```python
from build123d import *

# Parameters (mm, degrees)
BOSS_EXTRUDE1_DEPTH      = 2
BOSS_EXTRUDE2_DEPTH      = 1.7
BOSS_EXTRUDE2_DEPTH_BACK = 1.7
BOSS_EXTRUDE3_DEPTH      = 1.7
BOSS_EXTRUDE3_DEPTH_BACK = 1.7
BOSS_EXTRUDE4_DEPTH      = 1.7
BOSS_EXTRUDE4_DEPTH_BACK = 1.7
BOSS_EXTRUDE5_DEPTH      = 1.7
BOSS_EXTRUDE5_DEPTH_BACK = 1.7
SKETCH6_W                = 38.6
SKETCH6_H                = 47.5
CUT_EXTRUDE1_DEPTH       = 4
BOSS_EXTRUDE6_DEPTH      = 3.8
BOSS_EXTRUDE7_DEPTH      = 3.8
CUT_EXTRUDE2_DEPTH       = 20
CUT_EXTRUDE2_DEPTH_BACK  = 20
CUT_EXTRUDE3_DEPTH       = 11.15
CUT_EXTRUDE3_DEPTH_BACK  = 11.15
CUT_EXTRUDE4_DEPTH       = 11.15
CUT_EXTRUDE4_DEPTH_BACK  = 11.15
CUT_EXTRUDE5_DEPTH       = 16
CUT_EXTRUDE5_DEPTH_BACK  = 16
CUT_EXTRUDE6_DEPTH       = 16
CUT_EXTRUDE6_DEPTH_BACK  = 16


with BuildPart() as part:
    # Sketch1 → Boss-Extrude1 (new body)
    with BuildSketch(Plane.XY):
        with BuildLine():
            Line((-14.3, 18.25), (-14.3, -18.25))
            ThreePointArc((-14.3, -18.25), (-14.153553391, -18.603553391), (-13.8, -18.75))
            Line((-13.8, -18.75), (13.8, -18.75))
            ThreePointArc((13.8, -18.75), (14.153553391, -18.603553391), (14.3, -18.25))
            Line((14.3, -18.25), (14.3, 18.25))
            ThreePointArc((14.3, 18.25), (14.153553391, 18.603553391), (13.8, 18.75))
            Line((13.8, 18.75), (-13.8, 18.75))
            ThreePointArc((-13.8, 18.75), (-14.153553391, 18.603553391), (-14.3, 18.25))
        make_face()
    extrude(amount=BOSS_EXTRUDE1_DEPTH)

    # Sketch2 → Boss-Extrude2 (add, two sides)
    with BuildSketch(Plane.XY) as boss_extrude2_sk:
        with BuildLine():
            Line((-13.1, 12.5), (-10.1, 12.5))
            ThreePointArc((-10.1, 12.5), (-9.35, 13.25), (-10.1, 14))
            Line((-10.1, 14), (-13.1, 14))
            Line((-13.1, 14), (-13.1, 12.5))
        make_face()
    extrude(amount=BOSS_EXTRUDE2_DEPTH)
    extrude(boss_extrude2_sk.sketch, amount=-BOSS_EXTRUDE2_DEPTH_BACK)

    # Sketch3 → Boss-Extrude3 (add, two sides)
    with BuildSketch(Plane.XY) as boss_extrude3_sk:
        with BuildLine():
            Line((10.1, -14), (13.1, -14))
            Line((13.1, -14), (13.1, -12.5))
            Line((13.1, -12.5), (10.1, -12.5))
            ThreePointArc((10.1, -12.5), (9.35, -13.25), (10.1, -14))
        make_face()
    extrude(amount=BOSS_EXTRUDE3_DEPTH)
    extrude(boss_extrude3_sk.sketch, amount=-BOSS_EXTRUDE3_DEPTH_BACK)

    # Sketch4 → Boss-Extrude4 (add, two sides)
    with BuildSketch(Plane.XY) as boss_extrude4_sk:
        with BuildLine():
            Line((-13.1, -12.5), (-13.1, -14))
            Line((-13.1, -14), (-10.1, -14))
            ThreePointArc((-10.1, -14), (-9.35, -13.25), (-10.1, -12.5))
            Line((-10.1, -12.5), (-13.1, -12.5))
        make_face()
    extrude(amount=BOSS_EXTRUDE4_DEPTH)
    extrude(boss_extrude4_sk.sketch, amount=-BOSS_EXTRUDE4_DEPTH_BACK)

    # Sketch5 → Boss-Extrude5 (add, two sides)
    with BuildSketch(Plane.XY) as boss_extrude5_sk:
        with BuildLine():
            Line((10.1, 12.5), (13.1, 12.5))
            Line((13.1, 12.5), (13.1, 14))
            Line((13.1, 14), (10.1, 14))
            ThreePointArc((10.1, 14), (9.35, 13.25), (10.1, 12.5))
        make_face()
    extrude(amount=BOSS_EXTRUDE5_DEPTH)
    extrude(boss_extrude5_sk.sketch, amount=-BOSS_EXTRUDE5_DEPTH_BACK)

    # Sketch6 → Cut-Extrude1 (cut)
    with BuildSketch(Plane.XY.offset(-3)):
        Rectangle(SKETCH6_W, SKETCH6_H)
        with BuildLine():
            Line((-14.3, -4.045), (-11.298993595, -4.045))
            ThreePointArc((-11.298993595, -4.045), (-10.927421183, -4.210434697), (-10.801732648, -4.597264232))
            Line((-10.801732648, -4.597264232), (-11.79, -14))
            Line((-11.79, -14), (-8.55, -14))
            ThreePointArc((-8.55, -14), (-8.196446609, -14.146446609), (-8.05, -14.5))
            Line((-8.05, -14.5), (-8.05, -18.75))
            Line((-8.05, -18.75), (8.05, -18.75))
            Line((8.05, -18.75), (8.05, -14.5))
            ThreePointArc((8.05, -14.5), (8.196446609, -14.146446609), (8.55, -14))
            Line((8.55, -14), (11.79, -14))
            Line((11.79, -14), (10.801732648, -4.597264232))
            ThreePointArc((10.801732648, -4.597264232), (10.927421183, -4.210434697), (11.298993595, -4.045))
            Line((11.298993595, -4.045), (14.3, -4.045))
            Line((14.3, -4.045), (14.3, 4.045))
            Line((14.3, 4.045), (11.298993595, 4.045))
            ThreePointArc((11.298993595, 4.045), (10.927421183, 4.210434697), (10.801732648, 4.597264232))
            Line((10.801732648, 4.597264232), (11.79, 14))
            Line((11.79, 14), (8.55, 14))
            ThreePointArc((8.55, 14), (8.196446609, 14.146446609), (8.05, 14.5))
            Line((8.05, 14.5), (8.05, 18.75))
            Line((8.05, 18.75), (-8.05, 18.75))
            Line((-8.05, 18.75), (-8.05, 14.5))
            ThreePointArc((-8.05, 14.5), (-8.196446609, 14.146446609), (-8.55, 14))
            Line((-8.55, 14), (-11.79, 14))
            Line((-11.79, 14), (-10.801732648, 4.597264232))
            ThreePointArc((-10.801732648, 4.597264232), (-10.927421183, 4.210434697), (-11.298993595, 4.045))
            Line((-11.298993595, 4.045), (-14.3, 4.045))
            Line((-14.3, 4.045), (-14.3, -4.045))
        make_face(mode=Mode.SUBTRACT)
    extrude(amount=CUT_EXTRUDE1_DEPTH, mode=Mode.SUBTRACT)

    # Sketch7 → Boss-Extrude6 (add)
    with BuildSketch(Plane.XY.offset(-3.6)):
        Polygon((12.36, -4.002188077), (13.547735768, -15.302739052), (14.1, -15.8), (15.35, -15.8), (14.779051792, -11.15), (14.04, -11.15), (14.04, 11.15), (14.779051792, 11.15), (15.35, 15.8), (14.1, 15.8), (13.547735768, 15.302739052), (12.36, 4.002188077), align=None)
    extrude(amount=BOSS_EXTRUDE6_DEPTH)

    # Sketch8 → Boss-Extrude7 (add)
    with BuildSketch(Plane.XY.offset(-3.6)):
        Polygon((-15.35, -15.8), (-14.1, -15.8), (-13.547735768, -15.302739052), (-12.36, -4.002188077), (-12.36, 4.002188077), (-13.547735768, 15.302739052), (-14.1, 15.8), (-15.35, 15.8), (-14.779051792, 11.15), (-14.04, 11.15), (-14.04, -11.15), (-14.779051792, -11.15), align=None)
    extrude(amount=BOSS_EXTRUDE7_DEPTH)

    # Sketch9 → Cut-Extrude2 (cut, two sides)
    with BuildSketch(Plane(origin=(0, 0, 0), x_dir=(0, 0, -1), z_dir=(1, 0, 0))) as cut_extrude2_sk:
        Polygon((2.395156371, -15.8), (8.5, -15.8), (8.5, 15.8), (2.395156371, 15.8), (3.5, 0), align=None)
    extrude(amount=CUT_EXTRUDE2_DEPTH, mode=Mode.SUBTRACT)
    extrude(cut_extrude2_sk.sketch, amount=-CUT_EXTRUDE2_DEPTH_BACK, mode=Mode.SUBTRACT)

    # Sketch10 → Cut-Extrude3 (cut, two sides)
    with BuildSketch(Plane(origin=(0, 0, 0), x_dir=(1, 0, 0), z_dir=(0, 1, 0))) as cut_extrude3_sk:
        Polygon((13.602556682, 4), (14.04, -1), (14.3, -1), (14.3, 4), align=None)
    extrude(amount=CUT_EXTRUDE3_DEPTH, mode=Mode.SUBTRACT)
    extrude(cut_extrude3_sk.sketch, amount=-CUT_EXTRUDE3_DEPTH_BACK, mode=Mode.SUBTRACT)

    # Sketch11 → Cut-Extrude4 (cut, two sides)
    with BuildSketch(Plane(origin=(0, 0, 0), x_dir=(1, 0, 0), z_dir=(0, 1, 0))) as cut_extrude4_sk:
        Polygon((-14.3, 4), (-14.3, -1), (-14.04, -1), (-13.602556682, 4), align=None)
    extrude(amount=CUT_EXTRUDE4_DEPTH, mode=Mode.SUBTRACT)
    extrude(cut_extrude4_sk.sketch, amount=-CUT_EXTRUDE4_DEPTH_BACK, mode=Mode.SUBTRACT)

    # Sketch12 → Cut-Extrude5 (cut, two sides)
    with BuildSketch(Plane(origin=(0, 0, 0), x_dir=(1, 0, 0), z_dir=(0, 1, 0))) as cut_extrude5_sk:
        Polygon((12.35, 4.8), (12.35, 4.675260778), (15.35, 1.1), (15.35, 0.6), (14.375049256, 0.428089879), (14.43, -0.2), (17.35, -0.2), (17.35, 4.8), align=None)
    extrude(amount=CUT_EXTRUDE5_DEPTH, mode=Mode.SUBTRACT)
    extrude(cut_extrude5_sk.sketch, amount=-CUT_EXTRUDE5_DEPTH_BACK, mode=Mode.SUBTRACT)

    # Sketch13 → Cut-Extrude6 (cut, two sides)
    with BuildSketch(Plane(origin=(0, 0, 0), x_dir=(1, 0, 0), z_dir=(0, 1, 0))) as cut_extrude6_sk:
        Polygon((-17.35, 4.8), (-17.35, -0.2), (-14.43, -0.2), (-14.375049256, 0.428089879), (-15.35, 0.6), (-15.35, 1.1), (-12.35, 4.675260778), (-12.35, 4.8), align=None)
    extrude(amount=CUT_EXTRUDE6_DEPTH, mode=Mode.SUBTRACT)
    extrude(cut_extrude6_sk.sketch, amount=-CUT_EXTRUDE6_DEPTH_BACK, mode=Mode.SUBTRACT)


solid = part.part
```
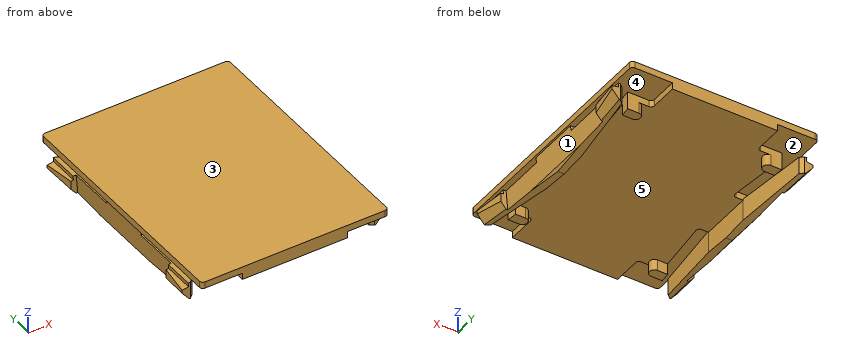
The model under review builds one solid part; all positions refer to its coordinate system, in mm. Face numbers are marked on the shaded views. A direction names the side the tool comes from. Coordinates: 2 decimals unless noted, no trailing zeros. Write each loop counter-clockwise with the first axis right and the second up, starting at its lowest first coordinate (ties: lowest second). Pieces come first, ordered by that corner, then holes. Notation, with made-up numbers: (-16, 6.5) - (11, 6.5) arc R6 cw to (11, 16.5) - close; hole circle Ø9 at (49.25, 25). An arc over 180 degrees is marked (long way). Answer in a Markdown table with one row per item. Add a question column.
Q1. To check wall thickness, follow line 1 along X through (y, z) = (-13, -0.6); line 2 along Y through (x, z) = (11, -0.15); line 3 along Z through (x, y) = (0, 1). State the ranges of each line that lie inside material, in increasing order. Write a range as from..to.
Q2. Consider section B-B on z = 1.4. Give the boundary of the cut face in (x, y).
Q3. Consider section C-C on x = -7.5. Give the boundary of the cut face in (y, z).
Q4. For the marked faces 1 and 2, list the 3-axis set-ups (+Z, -Z, +X, -X, +Y, -Y) from which the entire face can be reached by the end or side of a thin tool; tool diameter is ignored.
Q5. Consider section D-D on y = 13.25. Give the boundary of the cut face in (x, z), then the cut area to 3 significant figures.
Q6. Draft analysis for pull direction Z (two halves, no side actions). For the marked faces 3, 4 and 5, state which applies: +Z half, -Z half, draft (parallel to the pull), parting line (faces both ways), or undercut.
Q7. Clearance check with flat-ended pins moving along their axes: pin 1 (1 mm diameter, centred on y = -5, z = -1.5, fed in from +X) (3 decimals); pin 2 (0.5 mm diameter, centred on y = -17, z = 0.5, fed in from -X); pin 3 (0.6 mm diameter, centred on x = 15, z = -0.5, fed in from -Y); pin 4 (3 mm diameter, centred on x = 9.5, z = 0, fed in from +Y). State where each tip first meets the part, or that it passes through.
Q8. Consider section A-A on y = 8. Give the boundary of the cut face in (x, z), then the cut area to 3 significant figures.
Answers below:
| question | item | result |
|---|---|---|
| 1 | line 1 | -15.01..-13.31, -11.68..-9.39, 9.39..11.68, 13.31..15.01 |
| 1 | line 2 | -14..-12.5, 12.5..14 |
| 1 | line 3 | 0..2 |
| 2 | outline | (-14.3, -18.25) arc R0.5 ccw to (-13.8, -18.75) - (13.8, -18.75) arc R0.5 ccw to (14.3, -18.25) - (14.3, 18.25) arc R0.5 ccw to (13.8, 18.75) - (-13.8, 18.75) arc R0.5 ccw to (-14.3, 18.25) - close |
| 3 | outline | (-18.75, 0) - (18.75, 0) - (18.75, 2) - (-18.75, 2) - close |
| 4 | face 1 | -Z, +X |
| 4 | face 2 | -X |
| 5 | outline | (-15.04, -1.47) - (-14.11, -2.57) - (-13.33, -2.57) - (-13.33, 0.2) - (-14.43, 0.2) - (-14.38, -0.43) - (-15.04, -0.54) - close; (-14.3, 1) - (-11.71, 1) - (-11.71, -1.7) - (-9.35, -1.7) - (-9.35, 0) - (9.35, 0) - (9.35, -1.7) - (11.71, -1.7) - (11.71, 1) - (14.3, 1) - (14.3, 2) - (-14.3, 2) - close; (13.33, -2.57) - (14.11, -2.57) - (15.04, -1.47) - (15.04, -0.54) - (14.38, -0.43) - (14.43, 0.2) - (13.33, 0.2) - close |
| 5 | area | 67.6 mm² |
| 6 | face 3 | +Z half |
| 6 | face 4 | undercut |
| 6 | face 5 | -Z half |
| 7 | pin 1 | x = 13.865 |
| 7 | pin 2 | x = -8.05 |
| 7 | pin 3 | y = -15.8 |
| 7 | pin 4 | y = 18.75 |
| 8 | outline | (-14.3, 1) - (-11.16, 1) - (-11.16, 0) - (11.16, 0) - (11.16, 1) - (14.3, 1) - (14.3, 2) - (-14.3, 2) - close; (-13.97, 0.2) - (-13.7, -2.94) - (-12.78, -2.94) - (-12.78, 0.2) - close; (12.78, -2.94) - (13.7, -2.94) - (13.97, 0.2) - (12.78, 0.2) - close |
| 8 | area | 57.5 mm² |
